from build123d import *

# Parameters (mm, degrees)
F0_R     = 1.7859375
F1_DEPTH = 3.175


# Not quite as in the source:
# - a length typed as a fraction of an inch, garbled in the dataset ("3 / 203.2 mm" for 3/8 in), is restored


with BuildPart() as f1:
    # F0 (on Front) → F1 (new body)
    with BuildSketch(Plane.XZ):
        Polygon((75.715, -20), (75.715, 61.3500024), (-3.7115799668, 61.3500024), (-35.4027799668, 61.3500024), (-67.2774, 61.3500024), (-67.2774, -20), (-35.5862, -20), (-3.895, -20), align=None)
        with Locations((-63.3824, 0)):
            Circle(F0_R, mode=Mode.SUBTRACT)
        with Locations((-55.4124, 0)):
            Circle(F0_R, mode=Mode.SUBTRACT)
        with Locations((-47.4424, 0)):
            Circle(F0_R, mode=Mode.SUBTRACT)
        with Locations((-39.4724, 0)):
            Circle(F0_R, mode=Mode.SUBTRACT)
        with Locations((-31.7, 0)):
            Circle(F0_R, mode=Mode.SUBTRACT)
        with Locations((-23.73, 0)):
            Circle(F0_R, mode=Mode.SUBTRACT)
        with Locations((-15.76, 0)):
            Circle(F0_R, mode=Mode.SUBTRACT)
        with Locations((-7.79, 0)):
            Circle(F0_R, mode=Mode.SUBTRACT)
        Circle(F0_R, mode=Mode.SUBTRACT)
        with Locations((7.97, 0)):
            Circle(F0_R, mode=Mode.SUBTRACT)
        with Locations((15.94, 0)):
            Circle(F0_R, mode=Mode.SUBTRACT)
        with Locations((23.91, 0)):
            Circle(F0_R, mode=Mode.SUBTRACT)
        with Locations((31.88, 0)):
            Circle(F0_R, mode=Mode.SUBTRACT)
        with Locations((39.85, 0)):
            Circle(F0_R, mode=Mode.SUBTRACT)
        with Locations((47.82, 0)):
            Circle(F0_R, mode=Mode.SUBTRACT)
        with Locations((55.79, 0)):
            Circle(F0_R, mode=Mode.SUBTRACT)
        with Locations((63.76, 0)):
            Circle(F0_R, mode=Mode.SUBTRACT)
        with Locations((71.73, 0)):
            Circle(F0_R, mode=Mode.SUBTRACT)
        with Locations((-23.73, 40.005)):
            Circle(F0_R, mode=Mode.SUBTRACT)
    extrude(amount=F1_DEPTH)


solid = f1.part
Here's how the part is built. I have some questions about the finished solid (model axes, mm). Coordinates: 2 decimals unless noted, no trailing zeros. Order: outer loops, then holes, each group sorted by start corner. A loop starts at its lowest first (then second) coordinate and runs counter-clockwise, first axis right, second up. Notation, with made-up numbers: M -30.5,-10.75 L -14.5,-10.75 A23 ccw -14.5,20.25 Z; hole C 13,-37 d9. An arc over 180 degrees is marked long. Answer as CSV lines item,"result". Start each with the question number.
1. We'd pull the mould along Z, two halves only. Please class faces 1 (the cylindrical face through (-23.962, -1.565, 41.776)), 2 (the flat face through (3, -3.175, 21)): released by +Z, released by -Z, zero draft, split by the parting line, or undercut.
2. I want a section at A-A, the plane x = -7.79. Write out the boundary of the cut face in (y, z) (3 decimals).
3. I need wall thicknesses on line 1 (Z direction, x = -24, y = -2.9); line 2 (Z direction, x = -55.5, y = -1.4); line 3 (X direction, y = -2.4, z = 41) (3 decimals). Which ranges of each line are inside material? Lowest first, please. Write a range as [from, to].
4. I want a section at B-B, the plane y = -2.45. Count the separate pieces of the cut face and the enclosed holes in it, and give its area (3 significant figures).
Recorded:
1,face 1,"undercut"
1,face 2,"zero draft"
2,outline,"M -3.175,-20 L 0,-20 L 0,-1.786 L -3.175,-1.786 Z; M -3.175,1.786 L 0,1.786 L 0,61.35 L -3.175,61.35 Z"
3,line 1,"z = [-20, -1.77], [1.77, 38.24], [41.77, 61.35]"
3,line 2,"z = [-20, -1.78], [1.78, 61.35]"
3,line 3,"x = [-67.277, -25.213], [-22.247, 75.715]"
4,separate pieces,"1"
4,enclosed holes,"19"
4,area,"11,400 mm2"
